```python
from build123d import *

# Parameters (mm, degrees)
BOSS_EXTRUDE1_DEPTH     = 72
SKETCH4_R               = 19.05
CUT_EXTRUDE1_DEPTH      = 15
CUT_EXTRUDE2_DEPTH      = 280.154292263
CUT_EXTRUDE2_DEPTH_BACK = 72
FILLET2_R               = 5
FILLET3_R               = 5
SKETCH7_R               = 10
CUT_EXTRUDE3_DEPTH      = 20
CUT_EXTRUDE4_START      = -20
SKETCH8_R               = 10
CUT_EXTRUDE4_DEPTH      = 20
CUT_EXTRUDE5_DEPTH      = 62
CUT_EXTRUDE5_DEPTH_BACK = 266.891664466


with BuildPart() as part:
    # Sketch3 → Boss-Extrude1 (new body)
    with BuildSketch(Plane(origin=(0, 0, 0), x_dir=(0, 0, -1), z_dir=(1, 0, 0))):
        with BuildLine():
            Line((0, 0), (-100.313440323, 0))
            Line((-100.313440323, 0), (-142.357474116, -42.044033793))
            Line((-142.357474116, -42.044033793), (-142.357474116, -229.079611603))
            Line((-142.357474116, -229.079611603), (0, -229.079611603))
            ThreePointArc((0, -229.079611603), (-9.701802008, -156.011943225), (0, -82.944274847))
            Line((0, -82.944274847), (0, 0))
        make_face()
    extrude(amount=BOSS_EXTRUDE1_DEPTH)

    # Sketch4 → Cut-Extrude1 (cut)
    with BuildSketch(Plane(origin=(0, 0, 0), x_dir=(-1, 0, 0), z_dir=(0, 0, -1))):
        with Locations((-36, -41.472137424)):
            Circle(SKETCH4_R)
    extrude(amount=-CUT_EXTRUDE1_DEPTH, mode=Mode.SUBTRACT)

    # Sketch6 → Cut-Extrude2 (cut, two sides: drawn at the far end of the back side and taken through both)
    with BuildSketch(Plane.ZY.offset(-CUT_EXTRUDE2_DEPTH_BACK)):
        with BuildLine():
            Line((20, -194.079611603), (20, -229.079611603))
            Line((20, -229.079611603), (122.357474116, -229.079611603))
            Line((122.357474116, -229.079611603), (122.357474116, -194.079611603))
            ThreePointArc((122.357474116, -194.079611603), (120.893008022, -190.544077697), (117.357474116, -189.079611603))
            Line((117.357474116, -189.079611603), (25, -189.079611603))
            ThreePointArc((25, -189.079611603), (21.464466094, -190.544077697), (20, -194.079611603))
        make_face()
    extrude(amount=CUT_EXTRUDE2_DEPTH + CUT_EXTRUDE2_DEPTH_BACK, mode=Mode.SUBTRACT)

    # Fillet2
    fillet2_edges = [part.edges().sort_by_distance(p)[0] for p in [
        (36, -229.079611603, 122.357474116),
    ]]
    fillet(fillet2_edges, radius=FILLET2_R)

    # Fillet3
    fillet3_edges = [part.edges().sort_by_distance(p)[0] for p in [
        (36, -229.079611603, 20),
    ]]
    fillet(fillet3_edges, radius=FILLET3_R)

    # Sketch7 → Cut-Extrude3 (cut)
    with BuildSketch(Plane.XY.offset(20)):
        with Locations((36, -209.079611603)):
            Circle(SKETCH7_R)
    extrude(amount=-CUT_EXTRUDE3_DEPTH, mode=Mode.SUBTRACT)

    # Sketch8 → Cut-Extrude4 (cut)
    with BuildSketch(Plane(origin=(0, 0, 122.357474116), x_dir=(-1, 0, 0), z_dir=(0, 0, -1)).offset(CUT_EXTRUDE4_START)):
        with Locations(Location((-36, -209.079611603, 0), (0, 0, 180))):
            Circle(SKETCH8_R)
    extrude(amount=CUT_EXTRUDE4_DEPTH, mode=Mode.SUBTRACT)

    # 3DSketch1 → Cut-Extrude5 (cut, two sides: drawn at the far end of the back side and taken through both)
    with BuildSketch(Plane(origin=(0, -10, 10), x_dir=(0, -0.8328059611361112, 0.5535650197548234), z_dir=(1, 0, 0)).offset(-CUT_EXTRUDE5_DEPTH_BACK)):
        with BuildLine():
            Line((0, 0), (59.645268452, 39.646130972))
            add(Edge.make_bspline(
                [(59.645268452, 39.646130972), (59.851795376, 39.715600731), (60.058269091, 39.785227228), (60.264675078, 39.855053234), (63.229785209, 40.86201534), (66.17490971, 41.927849195), (68.900213672, 42.962126659), (76.587988483, 45.990190363), (84.19497116, 49.226232383), (89.073273504, 51.419920765), (100.476332318, 56.870903082), (111.513798328, 63.017783233), (117.769927201, 66.769037831), (127.427935538, 72.935642789), (136.853699774, 79.471867671), (140.230773606, 81.904573636), (143.55059138, 84.409472242), (146.799821395, 86.998315475)],
                knots=[0, 0, 0, 0, 0, 0, 0.010941255, 0.010941255, 0.010941255, 0.157238463, 0.157238463, 0.157238463, 0.425526751, 0.425526751, 0.425526751, 0.791499989, 0.791499989, 0.791499989, 1, 1, 1, 1, 1, 1], degree=5))
            add(Edge.make_bspline(
                [(146.799821395, 86.998315475), (146.838080386, 86.762713184), (146.881107812, 86.527938496), (146.928924899, 86.294146385), (147.096403086, 85.553769019), (147.312816425, 84.826481066), (147.482240174, 84.333957214), (147.795805007, 83.524872282), (148.156499747, 82.733389058), (148.30986597, 82.422264084), (148.555972143, 81.967326058), (148.831974102, 81.531039473), (148.925540772, 81.387965286), (149.020186904, 81.245580943), (149.114830616, 81.103195054), (149.115042333, 81.102876537)],
                knots=[0, 0, 0, 0, 0, 0, 0.186963411, 0.186963411, 0.186963411, 0.594974268, 0.594974268, 0.594974268, 0.865886461, 0.865886461, 0.865886461, 0.999699989, 1, 1, 1, 1, 1, 1], degree=5))
            Line((149.115042333, 81.102876537), (200.239850729, 4.188614121))
            add(Edge.make_bspline(
                [(200.239850729, 4.188614121), (200.33660104, 4.043058978), (200.433351351, 3.897503835), (200.531212292, 3.752716424), (200.831458899, 3.322960579), (201.161692533, 2.913933484), (201.392598415, 2.649392187), (201.990294831, 2.005724158), (202.622961514, 1.399585759), (203.015866658, 1.051305446), (203.829718887, 0.389334387), (204.702518346, -0.195889299), (205.152045635, -0.468884344), (206.074136833, -0.974780932), (207.035864281, -1.398770698), (207.525516965, -1.589737739), (208.520160048, -1.92851386), (209.540998156, -2.178769515), (210.056594039, -2.281493418), (211.095395611, -2.441585761), (212.14392909, -2.509871945), (212.669382635, -2.521145098), (213.720170989, -2.498114724), (214.765737187, -2.384257389), (215.285564899, -2.304395964), (216.311894633, -2.099178413), (217.313403497, -1.80116732), (217.805927348, -1.631743571), (218.615012281, -1.318178739), (219.406495505, -0.957483999), (219.717620478, -0.804117776), (220.172558504, -0.558011603), (220.608521923, -0.282214084), (220.751280697, -0.188863989), (220.89334807, -0.094431995), (221.035415443, 0)],
                knots=[0, 0, 0, 0, 0, 0, 0.037135909, 0.037135909, 0.037135909, 0.111407726, 0.111407726, 0.111407726, 0.222815452, 0.222815452, 0.222815452, 0.334223178, 0.334223178, 0.334223178, 0.445630904, 0.445630904, 0.445630904, 0.55703863, 0.55703863, 0.55703863, 0.668446357, 0.668446357, 0.668446357, 0.779854083, 0.779854083, 0.779854083, 0.890371964, 0.890371964, 0.890371964, 0.963753936, 0.963753936, 0.963753936, 1, 1, 1, 1, 1, 1], degree=5))
            Line((221.035415443, 0), (97.868875178, -81.868636245))
            Line((97.868875178, -81.868636245), (47.701419988, -71.763976232))
            Line((47.701419988, -71.763976232), (0, 0))
        make_face()
    extrude(amount=CUT_EXTRUDE5_DEPTH + CUT_EXTRUDE5_DEPTH_BACK, mode=Mode.SUBTRACT)


solid = part.part
```
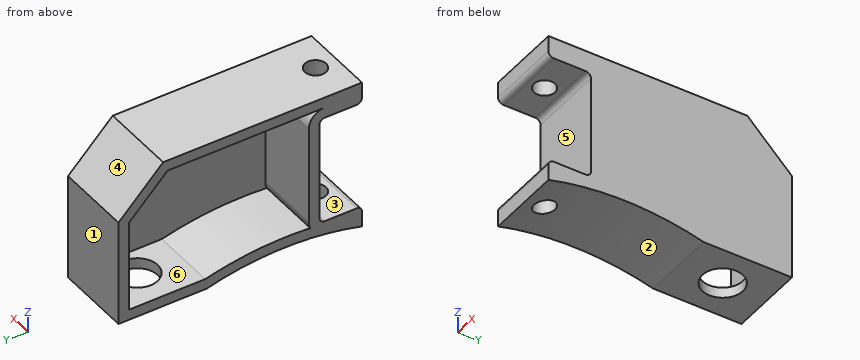
Geometry check sheet. Reference: the model listing, model coordinates, mm. Face numbers are marked on the shaded views. A direction names the side the tool comes from. Give positions to 0.01 mm unless a question says otherwise; leave off trailing zeros. Write each loop counter-clockwise with the first axis right and the second up, starting at its lowest first coordinate (ties: lowest second). Pieces come first, ordered by that corner, then holes. Notation, with made-up numbers: (83.5, 13.25) -> (142.5, 13.25) arc R30 ccw to (142.5, 37.25) -> close; hole circle Ø7 at (-10, -7.75). An arc over 180 degrees is marked (long way). Use one line per item in the form item = value.
Item 1: Sectioned sample at B-B on z = 39. Enter the section's corners in (x, y), plus the area to 3 significant figures.
Results list:
outline = (0, -189.08) -> (72, -189.08) -> (72, 0) -> (0, 0) -> (0, -10) -> (62, -10) -> (62, -179.08) -> (0, -179.08) -> close
area = 3,130 mm2
Item 2: Sectioned sample at C-C on x = 36. Count the separate pieces of the cut face and the enclosed holes in it, plus the area to 3 significant figures.
Results list:
separate_pieces = 3
enclosed_holes = 0
area = 6,210 mm2
Item 3: Mould release check, pull along Y, two halves, no side actions. Record for the marked faces 1, 2 and 3: released by +Y, released by -Y, zero draft, split by the parting line, or undercut.
Results list:
face_1 = released by +Y
face_2 = undercut
face_3 = zero draft
Item 4: Sectioned sample at A-A on x = 68. Enter the section's corners in (y, z).
Results list:
outline = (-229.08, 0) arc R280 cw to (-82.94, 0) -> (0, 0) -> (0, 100.31) -> (-42.04, 142.36) -> (-229.08, 142.36) -> (-229.08, 127.36) arc R5 ccw to (-224.08, 122.36) -> (-194.08, 122.36) arc R5 cw to (-189.08, 117.36) -> (-189.08, 25) arc R5 cw to (-194.08, 20) -> (-224.08, 20) arc R5 ccw to (-229.08, 15) -> close
Item 5: Depth check by flat-ended pin: pin 1 Ø1 at (x, y) = (13.5, -54.5) entering from -Z; pin 2 Ø9 at (x, y) = (53, -203) entering from -Z; pin 3 Ø10 at (x, z) = (61, 120.5) entering from +Y; pin 4 Ø10 at (x, y) = (40, -164.5) entering from -Z. Enter the tip coordinate at first touch or a pass-through.
Results list:
pin_1 = 0
pin_2 = 4.93
pin_3 = -15.19
pin_4 = 9.38
Item 6: Scan lines: line 1 (Y direction, x = 23, z = 58); line 2 (Z direction, x = 58, y = -119.5); line 3 (Z direction, x = 33, y = -87). Record each from-to range of solid material in increasing order.
Results list:
line_1 = -189.08 to -179.08, -10 to 0
line_2 = 7.31 to 17.39, 132.36 to 142.36
line_3 = 1.06 to 11.37, 132.36 to 142.36
Item 7: Access from +Z, -Z, +X, -X, +Y, -Y to the whole of each face (thin tool, end or side, straight path). Record for the marked faces 4, 5 and 6.
Results list:
face_4 = +Z, +X, -X, +Y
face_5 = +X, -X, -Y
face_6 = -X
